Build history of the part. All positions in model axes, mm. A direction names the side the tool comes from. Round coordinates to 2 decimals unless told otherwise and drop trailing zeros. Order: outer loops, then holes, each group sorted by start corner. A loop starts at its lowest first (then second) coordinate and runs counter-clockwise, first axis right, second up. Notation, with made-up numbers: M 66,-11 L 73,-11 A20 ccw 73,0 Z; hole C -6,41.5 d4. An arc over 180 degrees is marked long. Use CSV: the item, a comma, the result in double quotes.
from build123d import *

# Parameters (mm, degrees)
SKETCH1_R           = 2.1
SKETCH1_R_2         = 1.55
BOSS_EXTRUDE1_DEPTH = 4
BOSS_EXTRUDE2_DEPTH = 50
SKETCH3_R           = 2
SKETCH3_R_2         = 1
CUT_EXTRUDE1_DEPTH  = 10
FILLET1_R           = 3


with BuildPart() as part:
    # Sketch1 → Boss-Extrude1 (new body)
    with BuildSketch(Plane.XY):
        with BuildLine():
            Line((-7.842362425, 10.716234493), (-17.397624454, 40.071064625))
            ThreePointArc((-17.397624454, 40.071064625), (-25.795005306, 45.357497095), (-18.956793202, 38.167140452))
            Line((-18.956793202, 38.167140452), (-18.754238897, 37.544871045))
            Line((-18.754238897, 37.544871045), (-10.63810017, 12.611188123))
            Line((-10.63810017, 12.611188123), (-10.256851829, 11.439950722))
            ThreePointArc((-10.256851829, 11.439950722), (-11.874437039, 1.653788416), (-7.842362425, 10.716234493))
        make_face()
        with Locations((-10.438845238, 6.44326398)):
            Circle(SKETCH1_R, mode=Mode.SUBTRACT)
        with Locations((-21.926625837, 42.189589224)):
            Circle(SKETCH1_R_2, mode=Mode.SUBTRACT)
    boss_extrude1 = extrude(amount=BOSS_EXTRUDE1_DEPTH)

    # Sketch2 → Boss-Extrude2 (add)
    with BuildSketch(Plane.XY.offset(4)):
        Polygon((-16.14843876, 36.233426921), (-9.957962302, 17.215593153), (-7.105287237, 18.144164622), (-13.295763695, 37.161998389), align=None)
    extrude(amount=-BOSS_EXTRUDE2_DEPTH)

    # Mirror1: Boss-Extrude1 across plane
    add(boss_extrude1.mirror(Plane.XY.offset(-21)))

    # Sketch3 → Cut-Extrude1 (cut)
    with BuildSketch(Plane(origin=(-3.936983875, -1.281523768, 0), x_dir=(0, 0, 1), z_dir=(-0.950891688393093, -0.30952382290371966, 0))):
        with Locations(Location((-5, 34.452391, 0), (0, 0, 270))):
            Circle(SKETCH3_R)
        with Locations(Location((-5, 24.452391, 0), (0, 0, 90))):
            Circle(SKETCH3_R)
        with Locations(Location((-37, 24.452391, 0), (0, 0, 270))):
            Circle(SKETCH3_R)
        with Locations(Location((-37, 34.452391, 0), (0, 0, 90))):
            Circle(SKETCH3_R)
        with Locations(Location((-21, 29.452391, 0), (0, 0, 270))):
            Circle(SKETCH3_R_2)
    extrude(amount=-CUT_EXTRUDE1_DEPTH, mode=Mode.SUBTRACT)

    # Fillet1
    fillet1_edges = [part.edges().sort_by_distance(p)[0] for p in [
        (-9.957962302, 17.215593153, 2),
        (-9.957962302, 17.215593153, -44),
        (-16.14843876, 36.233426921, -44),
        (-16.14843876, 36.233426921, 2),
        (-10.256851829, 11.439950722, 2),
        (-7.842362425, 10.716234493, 2),
        (-7.842362425, 10.716234493, -44),
        (-10.256851829, 11.439950722, -44),
        (-17.397624454, 40.071064625, -44),
        (-18.956793202, 38.167140452, -44),
        (-17.397624454, 40.071064625, 2),
        (-18.956793202, 38.167140452, 2),
    ]]
    fillet(fillet1_edges, radius=FILLET1_R - 0.0001)  # a hair under: the kernel refuses the full size


solid = part.part
(1) Two-plate mould, pull along Z, no slides. Class faces 4 (the face through (-11.504, 26.744, -21.887)), 5 (the face through (-12.537, 6.536, -43.972)): released by +Z, released by -Z, zero draft, split by the parting line, or undercut.
Answer block:
face 4,"undercut"
face 5,"zero draft"
(2) Cut at D-D, the plane z = -38. Give the cut face in (x, y).
Answer block:
outline,"M -16.15,36.23 L -15.14,33.13 L -12.28,34.05 L -13.3,37.16 Z; M -14.06,29.83 L -12.04,23.62 L -9.19,24.55 L -11.21,30.76 Z; M -10.97,20.32 L -9.96,17.22 L -7.11,18.14 L -8.12,21.25 Z"
(3) Drop flat-ended pins along their axis: pin 1 (8 mm diameter, centred on y = 22, z = -22.5, fed in from -X); pin 2 (6 mm diameter, centred on y = 28.5, z = -19, fed in from +X). Give the stop position or say it passes through.
Answer block:
pin 1,"stops at x = -12.82"
pin 2,"stops at x = -9.5"
(4) Wall check: line 1 (Z direction, x = -18.75, y = 38.5); line 2 (Z direction, x = -11.25, y = 27); line 3 (X direction, y = 25, z = -37). Give the ranges that are in metal, low to high. Write a range as from..to.
Answer block:
line 1,"z = -46..-42, 0..4"
line 2,"z = -46..-21.96, -20.04..4"
line 3,"x = -12.49..-9.34"
(5) Tool access for faces 1 (the face through (-9.47, 25.41, -20.65)), 2 (the face through (-13.784, 28.971, -20.706)), 3 (the face through (-8.58, 12.98, -43.97)): list every direction of +Z, -Z, +X, -X, +Y, -Y with a clear straight run to the whole face (end or side of a thin tool).
Answer block:
face 1,"+Z, -Z, +X, +Y"
face 2,"-X, -Y"
face 3,"+Z, -Z, +X"
(6) Cut at B-B, the plane y = 5. Give the cut face in (x, z).
Answer block:
outline,"M -15.23,-46 L -11.96,-46 L -11.96,-42 L -15.23,-42 Z; M -15.23,0 L -11.96,0 L -11.96,4 L -15.23,4 Z; M -8.91,-46 L -5.65,-46 L -5.65,-42 L -8.91,-42 Z; M -8.91,0 L -5.65,0 L -5.65,4 L -8.91,4 Z"
(7) Cut at A-A, the plane y = 38.5. Give the cut face in (x, z).
Answer block:
outline,"M -25.3,-46 L -16.81,-46 L -16.81,-42 L -25.3,-42 Z; M -25.3,0 L -16.81,0 L -16.81,4 L -25.3,4 Z"
(8) Cut at C-C, the plane x = -22. Give the cut face in (y, z), and give its area (3 significant figures).
Answer block:
outline,"M 37.19,-46 L 40.64,-46 L 40.64,-42 L 37.19,-42 Z; M 37.19,0 L 40.64,0 L 40.64,4 L 37.19,4 Z; M 43.74,-46 L 47.19,-46 L 47.19,-42 L 43.74,-42 Z; M 43.74,0 L 47.19,0 L 47.19,4 L 43.74,4 Z"
area,"55.2 mm²"
